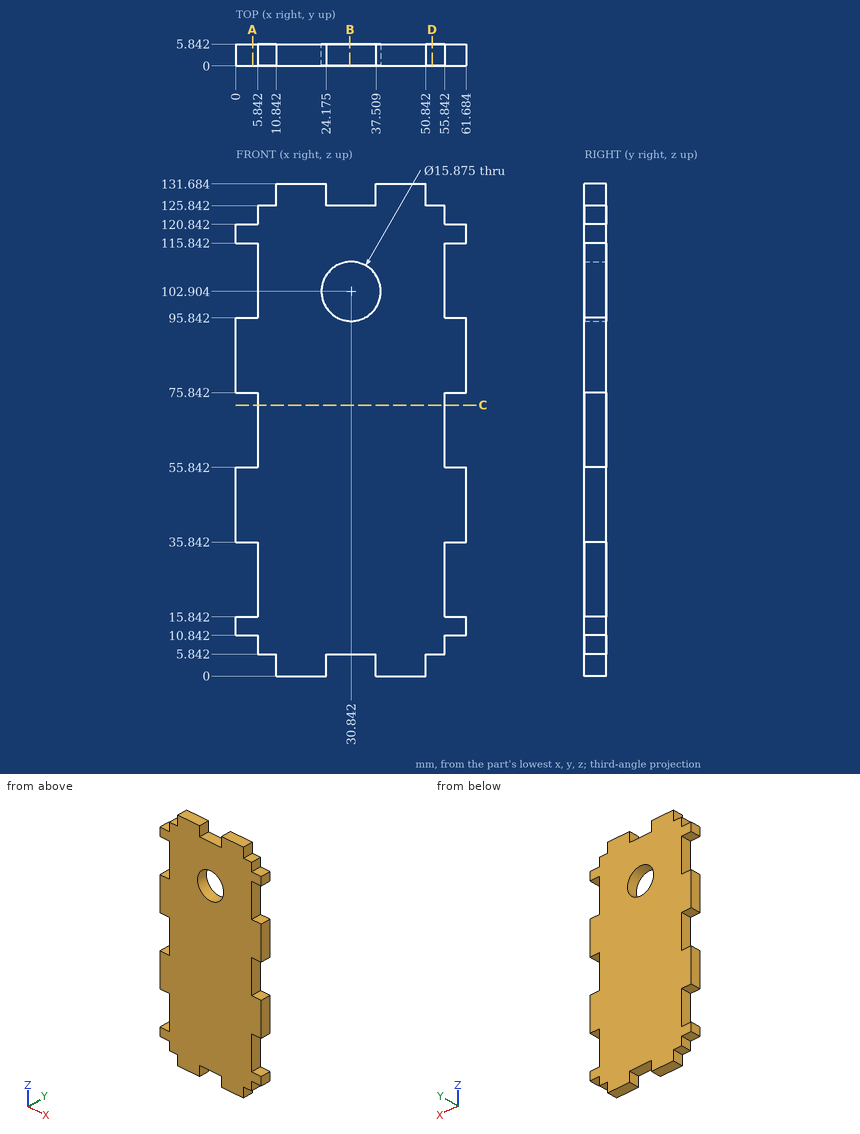
Drawing for the job (mm, zero at the part's lowest x, y, z). Round coordinates to 2 decimals unless told otherwise and drop trailing zeros. Loops run counter-clockwise (first coordinate to the right, second up) from the corner with the lowest first, then second, coordinate; pieces in that order, holes last. Notation, with made-up numbers: (58.25, -34.75) - (72.25, -34.75) arc R15 ccw to (72.25, -17.75) - close; hole circle Ø4 at (88.25, 29). An arc over 180 degrees is marked (long way). Return JSON: item names as keys, results as strings. Group by question number.
Q1. Band-saw the part on B-B on x = 30.5. Give the cut face in (y, z) (1 decimal).
Q2. Drill centre lines: line 1 along Z through (x, y) = (58, 1); line 2 along X through (y, z) = (3.7, 121); line 3 along Z through (x, y) = (9.5, 5.1). Where is each one in solid material? Low to high. Write a range as [from, to].
Q3. Flat gauge pins, fed straight in: pin 1 Ø1.8 at (y, z) = (3, 128) entering from -X; pin 2 Ø3 at (x, y) = (33.5, 2.5) entering from +Z; pin 3 Ø1.5 at (y, z) = (2, 124.5) entering from +X; pin 4 Ø5 at (x, z) = (32, 99) entering from -Y. Where does each tip first touch, or does it go through?
Q4. Band-saw the part on A-A on x = 4.5. Give the cut face in (y, z), plus the area to 3 significant figures.
Q5. Band-saw the part on D-D on x = 52.5. Give the cut face in (y, z), plus the area to 3 significant figures.
Q6. Band-saw the part on C-C on z = 72.5. Give the cut face in (x, y).
Solutions:
{
 "1": {"outline": "(0, 5.8) - (5.8, 5.8) - (5.8, 95) - (0, 95) - close; (0, 110.8) - (5.8, 110.8) - (5.8, 125.8) - (0, 125.8) - close"},
 "2": {"line 1": "z = [10.84, 15.84], [35.84, 55.84], [75.84, 95.84], [115.84, 120.84]", "line 2": "x = [5.84, 55.84]", "line 3": "z = [5.84, 125.84]"},
 "3": {"pin 1": "stops at x = 10.84", "pin 2": "stops at z = 125.84", "pin 3": "stops at x = 55.84", "pin 4": "passes through"},
 "4": {"outline": "(0, 10.84) - (5.84, 10.84) - (5.84, 15.84) - (0, 15.84) - close; (0, 35.84) - (5.84, 35.84) - (5.84, 55.84) - (0, 55.84) - close; (0, 75.84) - (5.84, 75.84) - (5.84, 95.84) - (0, 95.84) - close; (0, 115.84) - (5.84, 115.84) - (5.84, 120.84) - (0, 120.84) - close", "area": "292 mm^2"},
 "5": {"outline": "(0, 5.84) - (5.84, 5.84) - (5.84, 125.84) - (0, 125.84) - close", "area": "701 mm^2"},
 "6": {"outline": "(5.84, 0) - (55.84, 0) - (55.84, 5.84) - (5.84, 5.84) - close"}
}
